Could you check a few things on this model? Use its own coordinates, in mm. A direction names the side the tool comes from. Give positions to 0.01 mm unless a question says otherwise; leave off trailing zeros. Loops run counter-clockwise (first coordinate to the right, second up) from the corner with the lowest first, then second, coordinate; pieces in that order, holes last. Notation, with made-up numbers: M 33.5,10.25 L 82.5,10.25 A19 cw 82.5,33.25 Z; hole C -39,70 d7. An arc over 180 degrees is marked long. Return JSON: item names as keys, results as strings. Group by question number.
1. For pin 1 (1.4 mm diameter, centred on y = 1.5, z = 4, fed in from -X), with a flat end and sliding along its axis, tell me the tip position at first contact or that it passes through.
2. If we mould it in two halves opening along Y, with no side actions, what happens to faces 6 (the flat face through (9.9, 20, 0.3)), 7 (the flat face through (17, 13, 3)), 8 (the flat face through (13, 17, 3))? For each: +Y half, -Y half, draft (parallel to the pull), parting line (faces both ways), or undercut.
3. Please list where these lines run through material, in increasing order: line 1 (X direction, y = 2.75, z = 4); line 2 (X direction, y = 14.75, z = 3.9).
4. If we section it at B-B (x = 3.5): Write out the boundary of the cut face in (y, z), plus the area to 3 significant figures.
5. For faces 1 (the flat face through (17, 7, 3)), 2 (the flat face through (7, 17, 3)), 3 (the flat face through (6, 14, 3)), 4 (the flat face through (0, 9.9, 0.3)), 5 (the flat face through (16, 17, 5.6)), which set-ups out of +Z, -Z, +X, -X, +Y, -Y let a thin tool reach every point of the face, with its end or its side?
6. If we section it at D-D (x = 8.5): Write out the boundary of the cut face in (y, z), plus the area to 3 significant figures.
7. If we section it at A-A (z = 4.45): Write out the boundary of the cut face in (x, y).
```python
from build123d import *

# Parameters (mm, degrees)
BOX002_W     = 20
BOX002_H     = 6
BOX002_DEPTH = 10
BOX001_W     = 6
BOX001_H     = 20
BOX001_DEPTH = 10
BOX_W        = 20
BOX_H        = 20
BOX_DEPTH    = 4.6
CHAMFER_SIZE = 2
BOX003_W     = 20
BOX003_H     = 20
BOX003_DEPTH = 1


with BuildPart() as cube002:
    # Box002 → Box002 (new body)
    with BuildSketch(Plane(origin=(0, 7, 0), x_dir=(1, 0, 0), z_dir=(0, 0, 1))):
        with Locations((10, 3)):
            Rectangle(BOX002_W, BOX002_H)
    extrude(amount=BOX002_DEPTH)


with BuildPart() as fusion:
    # Box001 → Box001 (new body)
    with BuildSketch(Plane(origin=(7, 0, 0), x_dir=(1, 0, 0), z_dir=(0, 0, 1))):
        with Locations((3, 10)):
            Rectangle(BOX001_W, BOX001_H)
    extrude(amount=BOX001_DEPTH)

    # Fusion: union Cube002
    add(cube002.part)


with BuildPart() as base_button:
    # Box → Box (new body)
    with BuildSketch(Plane.XY):
        with Locations((10, 10)):
            Rectangle(BOX_W, BOX_H)
    extrude(amount=BOX_DEPTH)

    # Cut: cut Fusion
    add(fusion.part, mode=Mode.SUBTRACT)

    # Chamfer
    chamfer_edges = [base_button.edges().sort_by_distance(p)[0] for p in [
        (7, 7, 2.3),
        (7, 13, 2.3),
        (13, 13, 2.3),
        (13, 7, 2.3),
    ]]
    chamfer(chamfer_edges, length=CHAMFER_SIZE)


with BuildPart() as base_button_1:
    # Chamfer placement: moved
    add(base_button.part.moved(Location((0, 0, 1))))


with BuildPart() as single_pad_base:
    # Box003 → Box003 (new body)
    with BuildSketch(Plane.XY):
        with Locations((10, 10)):
            Rectangle(BOX003_W, BOX003_H)
    extrude(amount=BOX003_DEPTH)

    # Fusion001: union base_button
    add(base_button_1.part)


solid = single_pad_base.part
```
Answer:
{
 "1": {"pin 1": "stops at x = 0"},
 "2": {"face 6": "+Y half", "face 7": "undercut", "face 8": "draft"},
 "3": {"line 1": "x = 0 to 7, 13 to 20", "line 2": "x = 0 to 6.75, 13.25 to 20"},
 "4": {"outline": "M 0,0 L 20,0 L 20,5.6 L 13,5.6 L 13,1 L 7,1 L 7,5.6 L 0,5.6 Z", "area": "84.4 mm²"},
 "5": {"face 1": "+Z, +X, -X", "face 2": "+Z, +Y, -Y", "face 3": "+Z", "face 4": "+Z, -Z, -X, +Y, -Y", "face 5": "+Z, +X, -X, +Y, -Y"},
 "6": {"outline": "M 0,0 L 20,0 L 20,1 L 0,1 Z", "area": "20.0 mm²"},
 "7": {"outline": "M 0,0 L 7,0 L 7,5 L 5,7 L 0,7 Z; M 0,13 L 5,13 L 7,15 L 7,20 L 0,20 Z; M 13,0 L 20,0 L 20,7 L 15,7 L 13,5 Z; M 13,15 L 15,13 L 20,13 L 20,20 L 13,20 Z"}
}
